from build123d import *

# Parameters (mm, degrees)
SKETCH1_W           = 200
SKETCH1_H           = 30
BOSS_EXTRUDE1_DEPTH = 20
FILLET8_R           = 4
SKETCH3_W           = 13.877219135
SKETCH3_H           = 13.846786638
CUT_EXTRUDE1_DEPTH  = 200
SKETCH4_R           = 2
CUT_EXTRUDE2_DEPTH  = 20
SKETCH5_R           = 2
CUT_EXTRUDE3_DEPTH  = 20


with BuildPart() as part:
    # Sketch1 → Boss-Extrude1 (new body)
    with BuildSketch(Plane.XY):
        with Locations((10.755148741, -6.167048055)):
            Rectangle(SKETCH1_W, SKETCH1_H)
    extrude(amount=BOSS_EXTRUDE1_DEPTH)

    # Fillet8
    fillet8_edges = [part.edges().sort_by_distance(p)[0] for p in [
        (10.755148741, 8.832951945, 20),
        (10.755148741, 8.832951945, 0),
        (10.755148741, -21.167048055, 0),
        (10.755148741, -21.167048055, 20),
    ]]
    fillet(fillet8_edges, radius=FILLET8_R)

    # Sketch3 → Cut-Extrude1 (cut)
    with BuildSketch(Plane.ZY.offset(89.244851259)):
        with Locations((9.878270008, -10.893155572)):
            Rectangle(SKETCH3_W, SKETCH3_H)
    extrude(amount=-CUT_EXTRUDE1_DEPTH, mode=Mode.SUBTRACT)

    # Sketch4 → Cut-Extrude2 (cut)
    with BuildSketch(Plane(origin=(0, 8.832951945, 0), x_dir=(1, 0, 0), z_dir=(0, 1, 0))):
        with Locations((-84.647114684, -9.960432704)):
            Circle(SKETCH4_R)
    extrude(amount=-CUT_EXTRUDE2_DEPTH, mode=Mode.SUBTRACT)

    # Sketch5 → Cut-Extrude3 (cut)
    with BuildSketch(Plane(origin=(0, 8.832951945, 0), x_dir=(1, 0, 0), z_dir=(0, 1, 0))):
        with Locations((103.408272514, -9.882419894)):
            Circle(SKETCH5_R)
    extrude(amount=-CUT_EXTRUDE3_DEPTH, mode=Mode.SUBTRACT)


solid = part.part
Could you check a few things on this model? Use its own coordinates, in mm. A direction names the side the tool comes from. Coordinates: 2 decimals unless noted, no trailing zeros. Loops run counter-clockwise (first coordinate to the right, second up) from the corner with the lowest first, then second, coordinate; pieces in that order, holes last.
1. We'd pull the mould along Y, two halves only. Please class faces 4 (the face through (9, -17.817, 10)), 5 (the face through (9, -3.97, 10)), 6 (the face through (-86.645, 2.521, 9.872)), 7 (the face through (9, -21.167, 10)): released by +Y, released by -Y, zero draft, split by the parting line, or undercut.
2. I need wall thicknesses on L1, parallel to Y at x = 84.5, z = 9.5; L2, parallel to Z at x = -10, y = -4; L3, parallel to X at y = 0, z = 9.75. Which ranges of each line are inside material? Lowest first, please.
3. Imagine slicing it at A-A (y = -10). Please give me the cut outline in (x, z), and give its area (3 significant figures).
4. For faces 1 (the face through (101.934, 2.521, 8.531)), 2 (the face through (9, -6, 0)), 3 (the face through (9, -11, 2.94)), which set-ups out of +Z, -Z, +X, -X, +Y, -Y let a thin tool reach every point of the face, with its end or its side?
5. Imagine slicing it at B-B (x = 40.5). Please give me the cut outline in (y, z).
6. For P1, Ø3.5, axis at x = -84.65, z = 9.96, coming from the +Y side; P2, Ø5, axis at x = 103.41, z = 9.88, coming from the +Y side, each with a flat end and sliding along its axis, tell me the tip position at first contact or that it passes through.
Computed values:
1. face 4: undercut
1. face 5: undercut
1. face 6: zero draft
1. face 7: released by -Y
2. L1: y = -21.17 to -17.82, -3.97 to 8.83
2. L2: z = 0 to 2.94, 16.82 to 20
2. L3: x = -89.24 to -86.64, -82.66 to 101.41, 105.4 to 110.76
3. outline: (-89.24, 0) - (110.76, 0) - (110.76, 2.94) - (-89.24, 2.94) - close; (-89.24, 16.82) - (110.76, 16.82) - (110.76, 20) - (-89.24, 20) - close
3. area: 1,220 mm2
4. face 1: +Y
4. face 2: -Z, +X, -X, +Y, -Y
4. face 3: +X, -X
5. outline: (-21.17, 4) arc R4 ccw to (-17.17, 0) - (4.83, 0) arc R4 ccw to (8.83, 4) - (8.83, 16) arc R4 ccw to (4.83, 20) - (-17.17, 20) arc R4 ccw to (-21.17, 16) - close; hole (-17.82, 2.94) - (-3.97, 2.94) - (-3.97, 16.82) - (-17.82, 16.82) - close
6. P1: stops at y = -17.82
6. P2: stops at y = 8.83
